Input: part model. Units: mm. Frame: model coordinates. A direction names the side the tool comes from. Give positions to 0.01 mm unless a question says otherwise; leave off trailing zeros. Loops run counter-clockwise (first coordinate to the right, second up) from the corner with the lowest first, then second, coordinate; pieces in that order, holes last. Notation, with made-up numbers: (-38, 13.5) -> (-17, 13.5) arc R19 cw to (-17, 40.5) -> close; hole circle Ø9 at (18, 22). An arc over 180 degrees is marked (long way). Answer in a Markdown table with one row per item. Add a question column.
```python
from build123d import *

# Parameters (mm, degrees)
SKETCH2_W            = 90
SKETCH2_H            = 180
BOSS_EXTRUDE1_DEPTH  = 53
SKETCH3_W            = 80
SKETCH3_H            = 170
CUT_EXTRUDE1_DEPTH   = 49
SKETCH6_R            = 2.5
BOSS_EXTRUDE2_DEPTH  = 3
M2_CLEARANCE_HOLE1_D = 2.4
SKETCH17_W           = 5
SKETCH17_H           = 32
CUT_EXTRUDE8_DEPTH   = 29.5
SKETCH19_W           = 5
SKETCH19_H           = 13.5
CUT_EXTRUDE9_DEPTH   = 45
FILLET2_R            = 3
LPATTERN1_COUNT      = 2
LPATTERN1_PITCH      = 56
LPATTERN2_COUNT      = 2
LPATTERN2_PITCH      = 56
SKETCH29_W           = 11.5
SKETCH29_H           = 13.5
CUT_EXTRUDE12_DEPTH  = 10
LPATTERN4_COUNT      = 2
LPATTERN4_PITCH      = 112
SKETCH32_W           = 12.5
SKETCH32_H           = 11.5
CUT_EXTRUDE13_DEPTH  = 2
LPATTERN5_COUNT      = 3
LPATTERN5_PITCH      = 56
SKETCH33_W           = 8
SKETCH33_H           = 10
BOSS_EXTRUDE3_DEPTH  = 5.5
SKETCH34_W           = 3.5
SKETCH34_H           = 5
CUT_EXTRUDE14_DEPTH  = 8
SKETCH35_W           = 4
SKETCH35_H           = 10
CUT_EXTRUDE15_DEPTH  = 5.5
LPATTERN6_COUNT      = 3
LPATTERN6_PITCH      = 56
SKETCH36_R           = 7.375
CUT_EXTRUDE16_DEPTH  = 10
SKETCH24_R           = 1
CUT_EXTRUDE17_DEPTH  = 54


with BuildPart() as part:
    # Sketch2 → Boss-Extrude1 (new body)
    with BuildSketch(Plane.XY):
        Rectangle(SKETCH2_W, SKETCH2_H)
    extrude(amount=BOSS_EXTRUDE1_DEPTH)

    # Sketch3 → Cut-Extrude1 (cut)
    with BuildSketch(Plane.XY.offset(53)):
        Rectangle(SKETCH3_W, SKETCH3_H)
    extrude(amount=-CUT_EXTRUDE1_DEPTH, mode=Mode.SUBTRACT)

    # Sketch6 → Boss-Extrude2 (add)
    with BuildSketch(Plane.XY.offset(4)):
        with Locations((-23.7, 24.2)):
            Circle(SKETCH6_R)
        with Locations((-25, -24)):
            Circle(SKETCH6_R)
        with Locations((27.1, 9)):
            Circle(SKETCH6_R)
        with Locations((27.1, -18.9)):
            Circle(SKETCH6_R)
    boss_extrude2 = extrude(amount=BOSS_EXTRUDE2_DEPTH)

    # M2 Clearance Hole1 (through all)
    with Locations(Plane.XY.offset(7)):
        with Locations((-23.7, 24.2), (27.1, 9), (27.1, -18.9), (-25, -24)):
            m2_clearance_hole1 = Hole(M2_CLEARANCE_HOLE1_D / 2)

    # Sketch17 → Cut-Extrude8 (cut)
    with BuildSketch(Plane.XY.offset(53)):
        with Locations((-42.5, 6)):
            Rectangle(SKETCH17_W, SKETCH17_H)
    extrude(amount=-CUT_EXTRUDE8_DEPTH, mode=Mode.SUBTRACT)

    # Sketch19 → Cut-Extrude9 (cut)
    with BuildSketch(Plane.XY.offset(53)):
        with Locations((-42.5, 11.25)):
            Rectangle(SKETCH19_W, SKETCH19_H)
    extrude(amount=-CUT_EXTRUDE9_DEPTH, mode=Mode.SUBTRACT)

    # Fillet2
    fillet2_edges = [part.edges().sort_by_distance(p)[0] for p in [
        (-45, 90, 26.5),
        (45, 90, 26.5),
        (45, -90, 26.5),
        (-45, -90, 26.5),
    ]]
    fillet(fillet2_edges, radius=FILLET2_R)

    # LPattern1: Boss-Extrude2, M2 Clearance Hole1 ×2
    with Locations(*[(0, i * LPATTERN1_PITCH, 0) for i in range(1, LPATTERN1_COUNT)]):
        add(boss_extrude2)
        add(m2_clearance_hole1, mode=Mode.SUBTRACT)

    # LPattern2: Boss-Extrude2, M2 Clearance Hole1 ×2
    with Locations(*[(0, -i * LPATTERN2_PITCH, 0) for i in range(1, LPATTERN2_COUNT)]):
        add(boss_extrude2)
        add(m2_clearance_hole1, mode=Mode.SUBTRACT)

    # Sketch29 → Cut-Extrude12 (cut)
    with BuildSketch(Plane.ZY.offset(45)):
        with Locations((13.75, 67.25)):
            Rectangle(SKETCH29_W, SKETCH29_H)
    cut_extrude12 = extrude(amount=-CUT_EXTRUDE12_DEPTH, mode=Mode.SUBTRACT)

    # LPattern4: Cut-Extrude12 ×2
    with Locations(*[(0, -i * LPATTERN4_PITCH, 0) for i in range(1, LPATTERN4_COUNT)]):
        add(cut_extrude12, mode=Mode.SUBTRACT)

    # Sketch32 → Cut-Extrude13 (cut)
    with BuildSketch(Plane(origin=(-40, 0, 0), x_dir=(0, 0, -1), z_dir=(1, 0, 0))):
        with Locations((-14.25, 37.25)):
            Rectangle(SKETCH32_W, SKETCH32_H)
    cut_extrude13 = extrude(amount=-CUT_EXTRUDE13_DEPTH, mode=Mode.SUBTRACT)

    # LPattern5: Cut-Extrude13 ×3
    with Locations(*[(0, -i * LPATTERN5_PITCH, 0) for i in range(1, LPATTERN5_COUNT)]):
        add(cut_extrude13, mode=Mode.SUBTRACT)

    # Sketch33 → Boss-Extrude3 (add)
    with BuildSketch(Plane.ZY.offset(-40)):
        with Locations((38, -35)):
            Rectangle(SKETCH33_W, SKETCH33_H)
    boss_extrude3 = extrude(amount=BOSS_EXTRUDE3_DEPTH)

    # Sketch34 → Cut-Extrude14 (cut)
    with BuildSketch(Plane.XY.offset(42)):
        with Locations((38.25, -35)):
            Rectangle(SKETCH34_W, SKETCH34_H)
    cut_extrude14 = extrude(amount=-CUT_EXTRUDE14_DEPTH, mode=Mode.SUBTRACT)

    # Sketch35 → Cut-Extrude15 (cut)
    with BuildSketch(Plane.ZY.offset(-34.5)):
        with Locations((38, -35)):
            Rectangle(SKETCH35_W, SKETCH35_H)
    cut_extrude15 = extrude(amount=-CUT_EXTRUDE15_DEPTH, mode=Mode.SUBTRACT)

    # LPattern6: Boss-Extrude3, Cut-Extrude14, Cut-Extrude15 ×3
    with Locations(*[(0, i * LPATTERN6_PITCH, 0) for i in range(1, LPATTERN6_COUNT)]):
        add(boss_extrude3)
        add(cut_extrude14, mode=Mode.SUBTRACT)
        add(cut_extrude15, mode=Mode.SUBTRACT)

    # Sketch36 → Cut-Extrude16 (cut)
    with BuildSketch(Plane(origin=(0, 90, 0), x_dir=(1, 0, 0), z_dir=(0, 1, 0))):
        with Locations((15, -39)):
            Circle(SKETCH36_R)
    extrude(amount=-CUT_EXTRUDE16_DEPTH, mode=Mode.SUBTRACT)

    # Sketch24 → Cut-Extrude17 (cut, through all)
    with BuildSketch(Plane.XY.offset(53)):
        with Locations((-42.5, 87.5)):
            Circle(SKETCH24_R)
        with Locations((42.5, 87.5)):
            Circle(SKETCH24_R)
        with Locations((42.5, -87.5)):
            Circle(SKETCH24_R)
        with Locations((-42.5, -87.5)):
            Circle(SKETCH24_R)
        with Locations((-42.5, 27.5)):
            Circle(SKETCH24_R)
        with Locations((42.5, 27.5)):
            Circle(SKETCH24_R)
        with Locations((-42.5, -27.5)):
            Circle(SKETCH24_R)
        with Locations((42.5, -27.5)):
            Circle(SKETCH24_R)
    extrude(amount=-CUT_EXTRUDE17_DEPTH, mode=Mode.SUBTRACT)


solid = part.part
```
1) Section A-A on z = 49.5. State how many separate pieces and enclosed holes the cut face has, and give its area (3 significant figures).
2) Section B-B on x = 4.5. Output: boundary loops of the cut face in (y, z), and give its area (3 significant figures).
3) Material intervals for line 1 along X through (y, z) = (-87.5, 16); line 2 along X through (y, z) = (43, 7.5); line 3 along Y through (x, z) = (37.5, 48), sorted ascending.
4) Reachability of faces 4 (the face through (-43, 18, 16)), 5 (the face through (-25, -31, 7)), 6 (the face through (-42, -19, 14)) from +Z, -Z, +X, -X, +Y, -Y: full face, straight path, thin tool, end or side. Return the list, or none.
5) Pull-direction query (X, two-part tool) for faces 1 (the face through (-1, 1, 0)), 2 (the face through (28.44, -16.79, 5.48)), 3 (the face through (36, -35, 34)); classes: +X half, -X half, draft (parallel to the pull), parting line (faces both ways), or undercut.
6) Pin query (flat end, axial travel): pin 1 (2 mm diameter, centred on y = 19, z = 34.5, fed in from -X); pin 2 (1.6 mm diameter, centred on x = 36, y = -34.5, fed in from +Z); pin 3 (9 mm diameter, centred on x = 15, z = 39, fed in from +Y). Return the tip coordinate at first contact, or that it passes through.
Working result:
| question | item | result |
|---|---|---|
| 1 | separate pieces | 1 |
| 1 | enclosed holes | 8 |
| 1 | area | 2,410 mm2 |
| 2 | outline | (-90, 0) -> (90, 0) -> (90, 53) -> (85, 53) -> (85, 4) -> (-85, 4) -> (-85, 53) -> (-90, 53) -> close |
| 2 | area | 1,210 mm2 |
| 3 | line 1 | x = -44.96 to -43.5, -41.5 to 41.5, 43.5 to 44.96 |
| 3 | line 2 | x = -45 to -40, 40 to 45 |
| 3 | line 3 | y = -90 to -85, 85 to 90 |
| 4 | face 4 | +Z, -X |
| 4 | face 5 | +Z |
| 4 | face 6 | none |
| 5 | face 1 | draft |
| 5 | face 2 | undercut |
| 5 | face 3 | undercut |
| 6 | pin 1 | stops at x = 34.5 |
| 6 | pin 2 | stops at z = 42 |
| 6 | pin 3 | stops at y = -85 |
